Can you work these out from the model? Positions are in its coordinate system, mm. Round coordinates to 2 decimals unless told otherwise and drop trailing zeros. Loops run counter-clockwise (first coordinate to the right, second up) from the corner with the lowest first, then second, coordinate; pieces in that order, holes last.
```python
from build123d import *

# Parameters (mm, degrees)
CROQUIS1_W              = 5
CROQUIS1_H              = 350
SALIENTE_EXTRUIR1_DEPTH = 400
CROQUIS2_W              = 5
CROQUIS2_H              = 340
CROQUIS2_W_2            = 260.5
CROQUIS2_H_2            = 290
CROQUIS2_H_3            = 15
CORTAR_EXTRUIR1_DEPTH   = 30
CROQUIS3_R              = 3.175
CROQUIS3_R_2            = 3.05
CORTAR_EXTRUIR2_DEPTH   = 10


with BuildPart() as part:
    # Croquis1 → Saliente-Extruir1 (new body)
    with BuildSketch(Plane.XY):
        with Locations((-328.734660689, -84.960159363)):
            Rectangle(CROQUIS1_W, CROQUIS1_H)
    extrude(amount=-SALIENTE_EXTRUIR1_DEPTH)

    # Croquis2 → Cortar-Extruir1 (cut)
    with BuildSketch(Plane.ZY.offset(331.234660689)):
        with Locations((-112, -89.960159363)):
            Rectangle(CROQUIS2_W, CROQUIS2_H)
        with Locations((-254.75, -94.960159363)):
            Rectangle(CROQUIS2_W_2, CROQUIS2_H_2)
        with Locations((-397.5, 82.539840637)):
            Rectangle(CROQUIS2_W, CROQUIS2_H_3)
    extrude(amount=-CORTAR_EXTRUIR1_DEPTH, mode=Mode.SUBTRACT)

    # Croquis3 → Cortar-Extruir2 (cut)
    with BuildSketch(Plane.ZY.offset(331.234660689)):
        with Locations((-40.18483097, 60.17469511)):
            Circle(CROQUIS3_R)
        with Locations((-40.18483097, -232.010159363)):
            Circle(CROQUIS3_R_2)
    extrude(amount=-CORTAR_EXTRUIR2_DEPTH, mode=Mode.SUBTRACT)


solid = part.part
```
(1) Suppose I cut it at B-B (z = -217). Write out the boundary of the cut face in (x, y).
(2) Suppose I cut it at A-A (y = -158.5). Write out the boundary of the cut face in (x, z), then the cut area to 4 significant figures.
(3) If I drill on line 1 (Z direction, x = -328.7, y = -50); line 2 (Z direction, x = -330.3, y = 61); line 3 (Y direction, x = -329.35, z = -168.5), over which ranges is the centre line in solid material (lowest first)?
(4) Suppose I cut it at C-C (x = -328.15). Write out the boundary of the cut face in (y, z) (3 decimals), then the cut area to 3 significant figures.
(5) For pin 1 (1.5 mm diameter, centred on x = -328.5, z = -398.5, fed in from +Y), with a flat end and sliding along its axis, tell me the tip position at first contact or that it passes through.
Check result:
1. outline: (-331.23, -259.96) - (-326.23, -259.96) - (-326.23, -239.96) - (-331.23, -239.96) - close; (-331.23, 50.04) - (-326.23, 50.04) - (-326.23, 90.04) - (-331.23, 90.04) - close
2. outline: (-331.23, -400) - (-326.23, -400) - (-326.23, -385) - (-331.23, -385) - close; (-331.23, -124.5) - (-326.23, -124.5) - (-326.23, -114.5) - (-331.23, -114.5) - close; (-331.23, -109.5) - (-326.23, -109.5) - (-326.23, 0) - (-331.23, 0) - close
2. area: 672.5 mm2
3. line 1: z = -400 to -385, -124.5 to -114.5, -109.5 to 0
3. line 2: z = -400 to -114.5, -109.5 to -43.25, -37.12 to 0
3. line 3: y = -259.96 to -239.96, 50.04 to 90.04
4. outline: (-259.96, -400) - (75.04, -400) - (75.04, -395) - (90.04, -395) - (90.04, 0) - (-259.96, 0) - (-259.96, -109.5) - (80.04, -109.5) - (80.04, -114.5) - (-259.96, -114.5) - close; hole (-239.96, -385) - (50.04, -385) - (50.04, -124.5) - (-239.96, -124.5) - close; hole circle Ø6.1 at (-232.01, -40.185); hole circle Ø6.35 at (60.175, -40.185)
4. area: 62,600 mm2
5. pin 1: stops at y = 75.04
